from build123d import *

# Parameters (mm, degrees)
F0_W      = 144.2271173
F0_H      = 81.7665755749
F1_DEPTH  = 25.4
F2_W      = 96.966505982
F2_H      = 36.4053957164
F3_DEPTH  = 50.8
F4_OFFSET = 12.7


with BuildPart() as f1:
    # F0 (on Top) → F1 (new body)
    with BuildSketch(Plane.XY):
        with Locations((-1.0436475277, -7.1625672281)):
            Rectangle(F0_W, F0_H)
    extrude(amount=F1_DEPTH)


with BuildPart() as f3:
    # F2 (on Top) → F3 (new body)
    with BuildSketch(Plane.XY):
        with Locations((61.348229181, 35.0621510297)):
            Rectangle(F2_W, F2_H)
    extrude(amount=F3_DEPTH)

    # F4: cut F1, made larger all round first
    f4_tool = offset(f1.part, amount=F4_OFFSET, kind=Kind.INTERSECTION, mode=Mode.PRIVATE)
    add(f4_tool, mode=Mode.SUBTRACT)


solid = f3.part
Could you check a few things on this model? Use its own coordinates, in mm. A direction names the side the tool comes from. Give positions to 0.01 mm unless a question says otherwise; leave off trailing zeros. Order: outer loops, then holes, each group sorted by start corner. A loop starts at its lowest first (then second) coordinate and runs counter-clockwise, first axis right, second up. Notation, with made-up numbers: (88.5, 11) - (119.5, 11) arc R6 ccw to (119.5, 20) - close; hole circle Ø3 at (70, 8). An arc over 180 degrees is marked (long way). One line per question, with ' | ' between items. Start each with the question number.
Item 1: I want a section at A-A on y = 32.5. Write out the boundary of the cut face in (x, z), then the cut area to 3 significant figures.
Item 2: I want a section at B-B on z = 31. Write out the boundary of the cut face in (x, y).
Item 3: I'm going to push flat-ended pins straight in: pin 1 Ø10 at (x, z) = (59.5, 14) entering from -Y; pin 2 Ø9 at (y, z) = (30, 24) entering from -X. Where does each tip first touch, or does it pass through?
Item 4: For faces 1 (the flat face through (109.831, 35, 25)), 2 (the flat face through (48, 46.421, 19)), which set-ups out of +Z, -Z, +X, -X, +Y, -Y let a thin tool reach every point of the face, with its end or its side?
Item 5: I need wall thicknesses on probe 1 along Z at (x, y) = (37, 36); probe 2 along X at (y, z) = (42.5, 30); probe 3 along Y at (x, z) = (55.5, 33.5). Which ranges of each line are inside material? Lowest first, please. Write a range as [from, to].
Verdict:
1) outline: (12.86, 38.1) - (83.77, 38.1) - (83.77, 0) - (109.83, 0) - (109.83, 50.8) - (12.86, 50.8) - close | area: 2,220 mm^2
2) outline: (12.86, 46.42) - (83.77, 46.42) - (83.77, 16.86) - (109.83, 16.86) - (109.83, 53.26) - (12.86, 53.26) - close
3) pin 1: y = 46.42 | pin 2: x = 83.77
4) face 1: +Z, -Z, +X, +Y, -Y | face 2: -Z, -X, -Y
5) probe 1: [38.1, 50.8] | probe 2: [83.77, 109.83] | probe 3: [46.42, 53.26]
